Build history of the part. All positions in model axes, mm. A direction names the side the tool comes from. Round coordinates to 2 decimals unless told otherwise and drop trailing zeros. Loops run counter-clockwise (first coordinate to the right, second up) from the corner with the lowest first, then second, coordinate; pieces in that order, holes last. Notation, with made-up numbers: (-21, -11) - (21, -11) arc R30 ccw to (21, 25) - close; hole circle Ø1 at (-15.75, 84.25). An arc over 180 degrees is marked (long way). Put each result on its own line as item: value. Start each with the question number.
from build123d import *

# Parameters (mm, degrees)
F1_DEPTH = 5.08
F2_R     = 8.460003
F3_DEPTH = 25.4


with BuildPart() as f1:
    # F0 (on Top) → F1 (new body)
    with BuildSketch(Plane.XY):
        with BuildLine():
            ThreePointArc((10.689795, -2.593908), (10.922176, -1.306196), (11.000003, 0))
            ThreePointArc((11.000003, 0), (10.997729, 0.223701), (10.990905, 0.447309))
            ThreePointArc((10.990905, 0.447309), (10.93261, 1.215778), (10.820651, 1.978278))
            ThreePointArc((10.820651, 1.978278), (10.440932, 3.462227), (9.858754, 4.879041))
            ThreePointArc((9.858754, 4.879041), (9.492935, 5.557361), (9.080518, 6.208402))
            ThreePointArc((9.080518, 6.208402), (8.130051, 7.409612), (7.021935, 8.467143))
            ThreePointArc((7.021935, 8.467143), (6.411845, 8.938027), (5.770282, 9.365037))
            ThreePointArc((5.770282, 9.365037), (4.413411, 10.075807), (2.97096, 10.591198))
            ThreePointArc((2.97096, 10.591198), (2.222089, 10.773226), (1.462311, 10.902372))
            ThreePointArc((1.462311, 10.902372), (-0.066349, 10.999803), (-1.593721, 10.883939))
            ThreePointArc((-1.593721, 10.883939), (-2.351886, 10.745637), (-3.098507, 10.554588))
            ThreePointArc((-3.098507, 10.554588), (-4.534636, 10.021834), (-5.882834, 9.294748))
            ThreePointArc((-5.882834, 9.294748), (-6.519199, 8.860029), (-7.123565, 8.38182))
            ThreePointArc((-7.123565, 8.38182), (-8.218843, 7.310998), (-9.154751, 6.098411))
            ThreePointArc((-9.154751, 6.098411), (-9.559283, 5.442442), (-9.916893, 4.759758))
            ThreePointArc((-9.916893, 4.759758), (-10.481937, 3.336025), (-10.843728, 1.847603))
            ThreePointArc((-10.843728, 1.847603), (-10.946481, 1.083807), (-10.995501, 0.314692))
            ThreePointArc((-10.995501, 0.314692), (-10.93261, -1.215778), (-10.657726, -2.722672))
            ThreePointArc((-10.657726, -2.722672), (-10.440932, -3.462227), (-10.172887, -4.184788))
            ThreePointArc((-10.172887, -4.184788), (-9.492935, -5.557361), (-8.628907, -6.822173))
            ThreePointArc((-8.628907, -6.822173), (-8.130051, -7.409612), (-7.591288, -7.96068))
            ThreePointArc((-7.591288, -7.96068), (-6.411845, -8.938027), (-5.108071, -9.742058))
            ThreePointArc((-5.108071, -9.742058), (-4.413411, -10.075807), (-3.697086, -10.360098))
            ThreePointArc((-3.697086, -10.360098), (-2.222089, -10.773226), (-0.704003, -10.977452))
            ThreePointArc((-0.704003, -10.977452), (0.066349, -10.999803), (0.836375, -10.968161))
            ThreePointArc((0.836375, -10.968161), (2.351886, -10.745637), (3.821793, -10.314745))
            ThreePointArc((3.821793, -10.314745), (4.534636, -10.021834), (5.225219, -9.679729))
            ThreePointArc((5.225219, -9.679729), (6.519199, -8.860029), (7.686767, -7.868526))
            ThreePointArc((7.686767, -7.868526), (8.218843, -7.310998), (8.710576, -6.717584))
            ThreePointArc((8.710576, -6.717584), (9.559283, -5.442442), (10.222628, -4.061766))
            ThreePointArc((10.222628, -4.061766), (10.481937, -3.336025), (10.689795, -2.593908))
        make_face()
        with BuildLine():
            ThreePointArc((10.990905, 0.447309), (10.997729, 0.223701), (11.000003, 0))
            ThreePointArc((11.000003, 0), (10.922176, -1.306196), (10.689795, -2.593908))
            Line((10.689795, -2.593908), (13.474122, -1.334068))
            Line((13.474122, -1.334068), (10.990905, 0.447309))
        make_face()
        with BuildLine():
            ThreePointArc((9.858754, 4.879041), (10.440932, 3.462227), (10.820651, 1.978278))
            Line((10.820651, 1.978278), (12.851837, 4.261687))
            Line((12.851837, 4.261687), (9.858754, 4.879041))
        make_face()
        with BuildLine():
            Line((11.766608, -6.699151), (10.222628, -4.061766))
            ThreePointArc((10.222628, -4.061766), (9.559283, -5.442442), (8.710576, -6.717584))
            Line((8.710576, -6.717584), (11.766608, -6.699151))
        make_face()
        with BuildLine():
            ThreePointArc((7.021935, 8.467143), (8.130051, 7.409612), (9.080518, 6.208402))
            Line((9.080518, 6.208402), (10.007353, 9.120558))
            Line((10.007353, 9.120558), (7.021935, 8.467143))
        make_face()
        with BuildLine():
            Line((8.024541, -10.90589), (7.686767, -7.868526))
            ThreePointArc((7.686767, -7.868526), (6.519199, -8.860029), (5.225219, -9.679729))
            Line((5.225219, -9.679729), (8.024541, -10.90589))
        make_face()
        with BuildLine():
            ThreePointArc((2.97096, 10.591198), (4.413411, 10.075807), (5.770282, 9.365037))
            Line((5.770282, 9.365037), (5.432507, 12.402401))
            Line((5.432507, 12.402401), (2.97096, 10.591198))
        make_face()
        with BuildLine():
            Line((2.894958, -13.226901), (3.821793, -10.314745))
            ThreePointArc((3.821793, -10.314745), (2.351886, -10.745637), (0.836375, -10.968161))
            Line((0.836375, -10.968161), (2.894958, -13.226901))
        make_face()
        with BuildLine():
            ThreePointArc((-1.593721, 10.883939), (-0.066349, 10.999803), (1.462311, 10.902372))
            Line((1.462311, 10.902372), (-0.081669, 13.539757))
            Line((-0.081669, 13.539757), (-1.593721, 10.883939))
        make_face()
        with BuildLine():
            Line((-2.735189, -13.260861), (-0.704003, -10.977452))
            ThreePointArc((-0.704003, -10.977452), (-2.222089, -10.773226), (-3.697086, -10.360098))
            Line((-3.697086, -10.360098), (-2.735189, -13.260861))
        make_face()
        with BuildLine():
            ThreePointArc((-5.882834, 9.294748), (-4.534636, 10.021834), (-3.098507, 10.554588))
            Line((-3.098507, 10.554588), (-5.581724, 12.335966))
            Line((-5.581724, 12.335966), (-5.882834, 9.294748))
        make_face()
        with BuildLine():
            Line((-7.892398, -11.001898), (-5.108071, -9.742058))
            ThreePointArc((-5.108071, -9.742058), (-6.411845, -8.938027), (-7.591288, -7.96068))
            Line((-7.591288, -7.96068), (-7.892398, -11.001898))
        make_face()
        with BuildLine():
            ThreePointArc((-9.154751, 6.098411), (-8.218843, 7.310998), (-7.123565, 8.38182))
            Line((-7.123565, 8.38182), (-10.116648, 8.999174))
            Line((-10.116648, 8.999174), (-9.154751, 6.098411))
        make_face()
        with BuildLine():
            Line((-11.684939, -6.840606), (-8.628907, -6.822173))
            ThreePointArc((-8.628907, -6.822173), (-9.492935, -5.557361), (-10.172887, -4.184788))
            Line((-10.172887, -4.184788), (-11.684939, -6.840606))
        make_face()
        with BuildLine():
            ThreePointArc((-10.843728, 1.847603), (-10.481937, 3.336025), (-9.916893, 4.759758))
            Line((-9.916893, 4.759758), (-12.902311, 4.106343))
            Line((-12.902311, 4.106343), (-10.843728, 1.847603))
        make_face()
        with BuildLine():
            Line((-13.457048, -1.496512), (-10.657726, -2.722672))
            ThreePointArc((-10.657726, -2.722672), (-10.93261, -1.215778), (-10.995501, 0.314692))
            Line((-10.995501, 0.314692), (-13.457048, -1.496512))
        make_face()
    extrude(amount=F1_DEPTH)

    # F2 (on face) → F3 (cut)
    with BuildSketch(Plane.XY.offset(5.08)):
        Circle(F2_R)
    extrude(amount=-F3_DEPTH, mode=Mode.SUBTRACT)


solid = f1.part
Item 1: Slice it at B-B (y = -7.5). Give the cut face in (x, z).
Item 2: Which spindle directions (+Z, -Z, +X, -X, +Y, -Y) get a long thin tool onto all of the face, cutting with end or side? Do faces 1 (the flat face through (-12.21, -0.58, 2.5)), 2 (the flat face through (-6.52, -10.38, 2.5)), 3 (the flat face through (8.54, 8.8, 2.5)). Say none if no direction does.
Item 3: Drop flat-ended pins along their axis: pin 1 Ø1.5 at (y, z) = (-8.5, 4) entering from +X; pin 2 Ø3 at (y, z) = (8.5, 3) entering from +X; pin 3 Ø2 at (x, z) = (-2.5, 1.5) entering from -Y. Give the stop position or say it passes through.
Item 4: Two-plate mould, pull along Y, no slides. Class faces 4 (the cylindrical face through (0, -11, 3)), 5 (the flat face through (-12.08, -2.1, 2.5)), 6 (the flat face through (4.9, 7.2, 0)): pulls with the +Y half, pulls with the -Y half, needs draft (parallel to the pull), parting line crosses it, or undercut.
Item 5: Drill centre lines: probe 1 along X at (y, z) = (11, 3.75); probe 2 along Y at (x, z) = (-7.5, 3.7); probe 3 along X at (y, z) = (11.5, 2.95). Where is each one in solid material? Low to high. Write a range as [from, to].
Item 6: Slice it at A-A (y = 0). Give the cut face in (x, z).
Computed values:
1. outline: (-8.05, 0) - (-3.91, 0) - (-3.91, 5.08) - (-8.05, 5.08) - close; (3.91, 0) - (8.05, 0) - (8.05, 5.08) - (3.91, 5.08) - close
2. face 1: +Z, -Z, -X
2. face 2: +Z, -Z, -Y
2. face 3: +Z, -Z, +Y
3. pin 1: stops at x = 7.84
3. pin 2: stops at x = 10.01
3. pin 3: stops at y = -13.26
4. face 4: pulls with the -Y half
4. face 5: undercut
4. face 6: needs draft
5. probe 1: x = [-5.71, -3.72], [-1.53, 1.41], [3.53, 5.59]
5. probe 2: y = [-10.82, -3.91], [3.91, 8.46]
5. probe 3: x = [-5.66, -4.42], [-1.24, 1.11], [4.21, 5.53]
6. outline: (-11.42, 0) - (-8.46, 0) - (-8.46, 5.08) - (-11.42, 5.08) - close; (8.46, 0) - (11.61, 0) - (11.61, 5.08) - (8.46, 5.08) - close
